Build history of the part. All positions in model axes, mm. Face numbers are marked on the shaded views. Round coordinates to 2 decimals unless told otherwise and drop trailing zeros. Loops run counter-clockwise (first coordinate to the right, second up) from the corner with the lowest first, then second, coordinate; pieces in that order, holes last.
from build123d import *

# Parameters (mm, degrees)
BOSS_EXTRUDE1_DEPTH = 3
FILLET1_SIZE        = 2
FILLET1_SIZE_2      = 5
SKETCH2_R           = 3.05
SKETCH2_R_2         = 2.05
BOSS_EXTRUDE3_DEPTH = 9.5
SKETCH3_R           = 2.05
CUT_EXTRUDE1_DEPTH  = 44.548823309


with BuildPart() as part:
    # Sketch1 → Boss-Extrude1 (new body)
    with BuildSketch(Plane(origin=(0, 0, 0), x_dir=(1, 0, 0), z_dir=(0, 1, 0))):
        with BuildLine():
            Line((0, 6.5), (42, 6.5))
            Line((42, 6.5), (42, -6.5))
            Line((42, -6.5), (0, -6.5))
            ThreePointArc((0, -6.5), (-6.5, 0), (0, 6.5))
        make_face()
    extrude(amount=BOSS_EXTRUDE1_DEPTH)

    # Fillet1
    # an asymmetric fillet: 5, 2 mm, written as the material it takes off along each edge
    with BuildSketch(Plane(origin=(0, 0, -6.5), x_dir=(0, 1, 0), z_dir=(1, 0, 0)), Plane(origin=(54.5, 0, 6.5), x_dir=(0, 1, 0), z_dir=(-1, 0, 0))) as fillet1_piece_1:
        with BuildLine():
            Bezier((FILLET1_SIZE, 0), (0, 0), (0, FILLET1_SIZE_2), weights=[1, 0.707106781, 1])
            Line((0, FILLET1_SIZE_2), (0, 0))
            Line((0, 0), (FILLET1_SIZE, 0))
        make_face()
    extrude(amount=54.5, mode=Mode.SUBTRACT)
    with BuildSketch(Plane(origin=(0, 0, 0), x_dir=(0, 0, 1), z_dir=(1, 0, 0))) as fillet1_piece_2:
        with BuildLine():
            Bezier((6.5, -FILLET1_SIZE), (6.5, 0), (6.5 - FILLET1_SIZE_2, 0), weights=[1, 0.707106781, 1])
            Line((6.5 - FILLET1_SIZE_2, 0), (6.5, 0))
            Line((6.5, 0), (6.5, -FILLET1_SIZE))
        make_face()
    revolve(axis=Axis((0, 0, 0), (0, -1, 0)), revolution_arc=180, mode=Mode.SUBTRACT)

    # Sketch2 → Boss-Extrude3 (add)
    with BuildSketch(Plane(origin=(0, 3, 0), x_dir=(1, 0, 0), z_dir=(0, 1, 0))):
        with Locations(Location((0, 0, 0), (0, 0, 270))):
            Circle(SKETCH2_R)
        with Locations(Location((0, 0, 0), (0, 0, 270))):
            Circle(SKETCH2_R_2, mode=Mode.SUBTRACT)
    extrude(amount=-BOSS_EXTRUDE3_DEPTH)

    # Sketch3 → Cut-Extrude1 (cut, through all)
    with BuildSketch(Plane(origin=(0, 3, 0), x_dir=(1, 0, 0), z_dir=(0, 1, 0))):
        with Locations(Location((0, 0, 0), (0, 0, 270))):
            Circle(SKETCH3_R)
    extrude(amount=-CUT_EXTRUDE1_DEPTH, mode=Mode.SUBTRACT)


solid = part.part
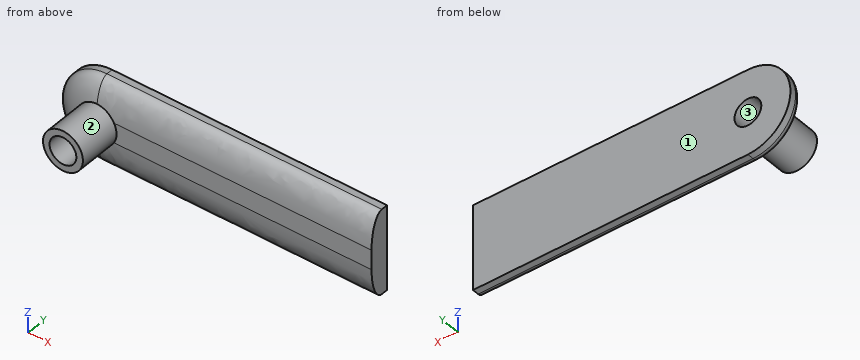
(1) Pull direction Z, two halves, no side cores. Call the marked faces 1, 2 and 3: +Z half, -Z half, draft (parallel to the pull), parting line (faces both ways), or undercut.
Responses:
face 1: draft
face 2: parting line
face 3: undercut
(2) Slice it at A-A on y = -3.5. List the corners of the cut face in (x, z), plus the area to 3 significant figures.
Responses:
outline: circle Ø6.1 at (0, 0); hole circle Ø4.1 at (0, 0)
area: 16.0 mm2
(3) Pin check, flat tips, straight feed: P1, Ø5, axis at y = 1.5, z = 4, coming from the -X side; P2, Ø0.9, axis at x = 31, z = -0.5, coming from the -Y side; P3, Ø4, axis at y = -2, z = -4.5, coming from the -X side. Stop position of each tip, or through.
Responses:
P1: stops at x = -6.31
P2: stops at y = 0
P3: stops at x = -1.75
(4) Probe line 1 (X direction, y = -3.75, z = 0); line 2 (Y direction, x = 28, z = 3); line 3 (X direction, y = 0.75, z = 0). List the from-to ranges inside material, lowest first.
Responses:
line 1: x = -3.05 to -2.05, 2.05 to 3.05
line 2: y = 0.09 to 3
line 3: x = -5.4 to -2.05, 2.05 to 42
